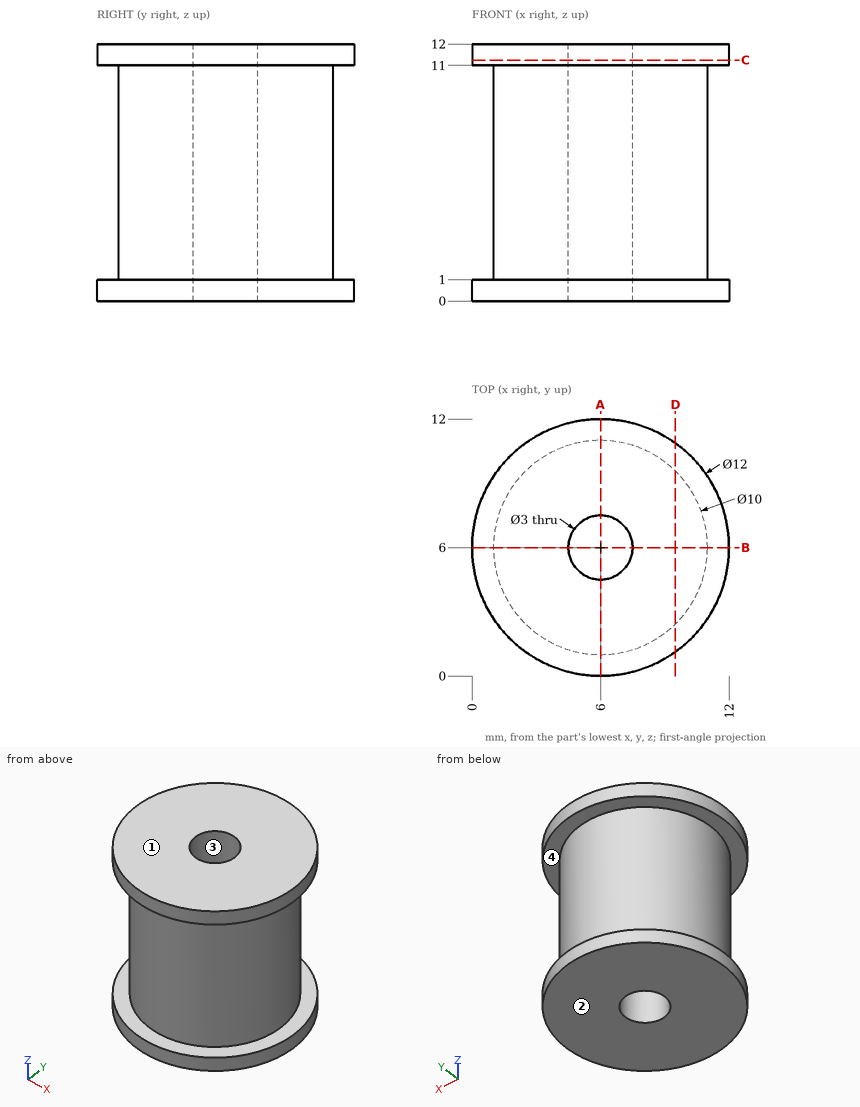
The figure shows three views and two pictorial views of one solid part (mm, origin at its lowest corner). Answer the questions. Give positions to 0.01 mm unless a question says otherwise; leave off trailing zeros. Loops run counter-clockwise (first coordinate to the right, second up) from the corner with the lowest first, then second, coordinate; pieces in that order, holes last. Notation, with made-up numbers: (39.25, 48) -> (76.25, 48) arc R20 cw to (76.25, 69) -> close; hole circle Ø7 at (78, 67). An arc over 180 degrees is marked (long way). Put each result on its own line as item: value. Start each with the question number.
Item 1: The mould has two halves that part along Z. Classify the marked faces 1, 2, 3 and 4: released by +Z, released by -Z, zero draft, split by the parting line, or undercut.
Item 2: Each of these flat-tipped pins is pushed along its axis until it touches: P1, Ø1.5, axis at y = 2, z = 8.5, coming from the +X side; P2, Ø1.5, axis at y = 10.5, z = 7.5, coming from the +X side; P3, Ø6, axis at x = 10.5, z = 8.5, coming from the -Y side; P4, Ø2.5, axis at x = 6, y = 6, coming from the -Z side. Where does it stop, or does it pass through?
Item 3: The part is cut by section D-D (x = 9.5). Give the vertices of the cut face in (y, z), then the cut area to 3 significant figures.
Item 4: Find the intervals of material crossed by L1, parallel to Z at x = 1, y = 3; L2, parallel to Y at x = 6, z = 7.5; L3, parallel to X at y = 5.75, z = 11.75, in increasing order. Write a range as [from, to].
Item 5: The part is cut by section C-C (z = 11.25). Give the vertices of the cut face in (x, y), then the cut area to 3 significant figures.
Item 6: The part is cut by section A-A (x = 6). Give the vertices of the cut face in (y, z), then the cut area to 3 significant figures.
Answers below:
1. face 1: released by +Z
1. face 2: released by -Z
1. face 3: zero draft
1. face 4: undercut
2. P1: x = 9.8
2. P2: x = 9.31
2. P3: y = 0.72
2. P4: through
3. outline: (1.13, 0) -> (10.87, 0) -> (10.87, 1) -> (9.57, 1) -> (9.57, 11) -> (10.87, 11) -> (10.87, 12) -> (1.13, 12) -> (1.13, 11) -> (2.43, 11) -> (2.43, 1) -> (1.13, 1) -> close
3. area: 90.9 mm2
4. L1: [0, 1], [11, 12]
4. L2: [1, 4.5], [7.5, 11]
4. L3: [0.01, 4.52], [7.48, 11.99]
5. outline: circle Ø12 at (6, 6); hole circle Ø3 at (6, 6)
5. area: 106 mm2
6. outline: (0, 0) -> (4.5, 0) -> (4.5, 12) -> (0, 12) -> (0, 11) -> (1, 11) -> (1, 1) -> (0, 1) -> close; (7.5, 0) -> (12, 0) -> (12, 1) -> (11, 1) -> (11, 11) -> (12, 11) -> (12, 12) -> (7.5, 12) -> close
6. area: 88.0 mm2
